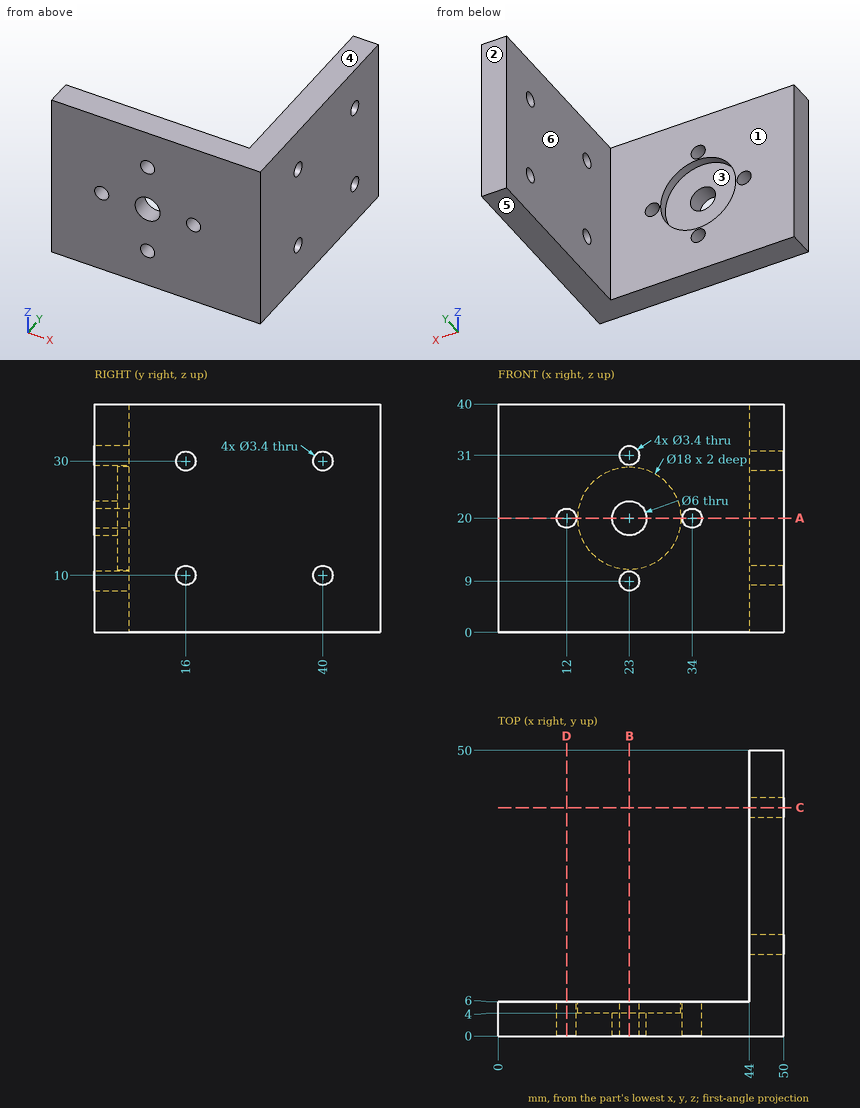
Input: dimensioned drawing with shaded views. Units: mm. Origin: part minimum x, y, z. A direction names the side the tool comes from. Give positions to 0.01 mm unless a question says otherwise; leave off trailing zeros. Write each loop counter-clockwise with the first axis right and the second up, starting at its lowest first coordinate (ties: lowest second). Pieces come first, ordered by that corner, then holes.
Q1. First-contact query: P1, Ø12, axis at y = 38, z = 23, coming from the -X side; P2, Ø4.5, axis at x = 34, z = 20, coming from the +Y side. Flat tips, straight axial feed; report the tip coordinate or a pass-through.
Q2. Material intervals for probe 1 along X at (y, z) = (2.3, 20); probe 2 along Z at (x, y) = (45.5, 16); probe 3 along X at (y, z) = (31.5, 8), sorted ascending.
Q3. Section D-D, the plane x = 12. Output: boundary loops of the cut face in (y, z).
Q4. Pull-direction query (Z, two-part tool) for the marked faces 3, 4, 5 and 6; classes: pulls with the +Z half, pulls with the -Z half, needs draft (parallel to the pull), parting line crosses it, or undercut.
Q5. Section C-C, the plane y = 40. Output: boundary loops of the cut face in (x, z), plus the area to 3 significant figures.
Q6. Set-up query: the marked faces 1 and 2. Return all of +Z, -Z, +X, -X, +Y, -Y with unobstructed straight access to the full face (end or side cutting, diameter ignored); none if empty.
Q7. Section B-B, the plane x = 23. Output: boundary loops of the cut face in (y, z).
Q8. Section A-A, the plane z = 20. Output: boundary loops of the cut face in (x, y).
Filled in:
1. P1: stops at x = 44
1. P2: stops at y = 6
2. probe 1: x = 0 to 10.3, 13.7 to 20, 26 to 32.3, 35.7 to 50
2. probe 2: z = 0 to 8.3, 11.7 to 28.3, 31.7 to 40
2. probe 3: x = 44 to 50
3. outline: (0, 0) - (6, 0) - (6, 18.3) - (0, 18.3) - close; (0, 21.7) - (6, 21.7) - (6, 40) - (0, 40) - close
4. face 3: undercut
4. face 4: pulls with the +Z half
4. face 5: pulls with the -Z half
4. face 6: needs draft
5. outline: (44, 0) - (50, 0) - (50, 8.3) - (44, 8.3) - close; (44, 11.7) - (50, 11.7) - (50, 28.3) - (44, 28.3) - close; (44, 31.7) - (50, 31.7) - (50, 40) - (44, 40) - close
5. area: 199 mm2
6. face 1: +Z, -Z, -X, +Y
6. face 2: +Z, -Z, +X, -X, +Y
7. outline: (0, 0) - (6, 0) - (6, 7.3) - (0, 7.3) - close; (0, 10.7) - (6, 10.7) - (6, 11) - (4, 11) - (4, 17) - (0, 17) - close; (0, 23) - (4, 23) - (4, 29) - (6, 29) - (6, 29.3) - (0, 29.3) - close; (0, 32.7) - (6, 32.7) - (6, 40) - (0, 40) - close
8. outline: (0, 0) - (10.3, 0) - (10.3, 6) - (0, 6) - close; (13.7, 0) - (20, 0) - (20, 4) - (14, 4) - (14, 6) - (13.7, 6) - close; (26, 0) - (32.3, 0) - (32.3, 6) - (32, 6) - (32, 4) - (26, 4) - close; (35.7, 0) - (50, 0) - (50, 50) - (44, 50) - (44, 6) - (35.7, 6) - close
